Can you work these out from the model? Positions are in its coordinate system, mm. Face numbers are marked on the shaded views. A direction names the side the tool comes from. Give positions to 0.01 mm unless a question says otherwise; leave off trailing zeros. Order: outer loops, then holes, each group sorted by start corner. A loop starts at its lowest first (then second) coordinate and runs counter-clockwise, first axis right, second up. Notation, with made-up numbers: M -24.5,10.25 L 14.5,10.25 A24 ccw 14.5,33.25 Z; hole C 34.25,-16 d1. An arc over 180 degrees is marked long. One line per question, with ' | ' between items. Start each with the question number.
1) If we section it at A-A, the plane y = 7: Please give me the cut outline in (x, z), plus the area to 3 significant figures.
2) I'm going to push flat-ended pins straight in: pin 1 Ø6 at (x, y) = (-20.5, 0) entering from -Z; pin 2 Ø12 at (x, z) = (-54, -16.5) entering from +Y; pin 3 Ø6 at (y, z) = (29, -5.5) entering from +X. Where does each tip first touch, or does it pass through?
3) If we section it at B-B, the plane x = -31: Please give me the cut outline in (y, z).
4) For the marked faces 1 and 2, which set-ups out of +Z, -Z, +X, -X, +Y, -Y let a thin tool reach every point of the face, with its end or its side?
5) Please list where these lines run through material, in increasing order: line 1 along Y through (x, z) = (-44, -14.75); line 2 along Z through (x, y) = (-12.5, -12); line 3 along Y through (x, z) = (-53, -1). Write a range as [from, to].
6) If we section it at D-D, the plane x = -5: Please give me the cut outline in (y, z).
7) If we section it at C-C, the plane z = -15.25: Please give me the cut outline in (x, y).
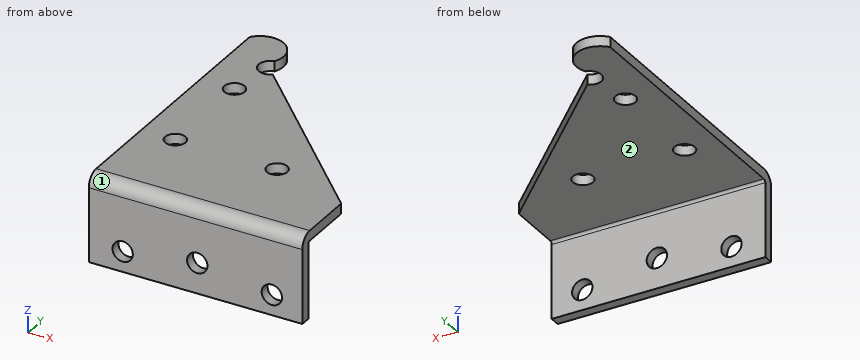
```python
from build123d import *

# Parameters (mm, degrees)
SCHIZZO2_R                           = 3
BASE_FLANGIA1_DEPTH                  = 3
PIEGATURA_START                      = -41.4
PIEGATURA_DELLO_SCHIZZO1_OUTLINE_W   = 63
PIEGATURA_DELLO_SCHIZZO1_OUTLINE_H   = 3
PIEGATURA_DELLO_SCHIZZO1_DEPTH       = 21.6634
PIEGATURA_START_2                    = -19.383939692
PIEGATURA_DELLO_SCHIZZO1_2_OUTLINE_W = 63
PIEGATURA_DELLO_SCHIZZO1_2_OUTLINE_H = 22.623356935
PIEGATURA_DELLO_SCHIZZO1_2_OUTLINE_R = 3
PIEGATURA_DELLO_SCHIZZO1_2_DEPTH     = 2.647339692
PIEGATURA_START_3                    = -19.7366
PIEGATURA_DELLO_SCHIZZO1_3_OUTLINE_W = 63
PIEGATURA_DELLO_SCHIZZO1_3_OUTLINE_H = 22.623356935
PIEGATURA_DELLO_SCHIZZO1_3_OUTLINE_R = 3
PIEGATURA_DELLO_SCHIZZO1_3_DEPTH     = 3.7366
PIEGATURA_START_4                    = -64
PIEGATURA_DELLO_SCHIZZO1_4_DEPTH     = 64


with BuildPart() as part:
    # Base-Flangia1: sheet metal written as solids
    # Schizzo2 → Base-Flangia1 (new body)
    with BuildSketch(Plane.XY):
        with BuildLine():
            Line((0, 0), (0, -41.4))
            Line((0, -41.4), (-63, -41.4))
            Line((-63, -41.4), (-63, 61.925683224))
            ThreePointArc((-63, 61.925683224), (-53.724596428, 63.490157792), (-51.266546346, 54.410582808))
            ThreePointArc((-51.266546346, 54.410582808), (-53.647048092, 49.463861618), (-48.285339065, 48.285339065))
            Line((-48.285339065, 48.285339065), (0, 0))
        make_face()
        with Locations((-53, 37)):
            Circle(SCHIZZO2_R, mode=Mode.SUBTRACT)
        with Locations((-53, 7)):
            Circle(SCHIZZO2_R, mode=Mode.SUBTRACT)
        with Locations((-23, 7)):
            Circle(SCHIZZO2_R, mode=Mode.SUBTRACT)
        with Locations((-53, -35.4)):
            Circle(SCHIZZO2_R, mode=Mode.SUBTRACT)
        with Locations((-31, -32.4)):
            Circle(SCHIZZO2_R, mode=Mode.SUBTRACT)
        with Locations((-9, -35.4)):
            Circle(SCHIZZO2_R, mode=Mode.SUBTRACT)
    extrude(amount=-BASE_FLANGIA1_DEPTH)

    # Piegatura dello schizzo1: read off the stored shape, not the designer's step
    # Piegatura dello schizzo1 outline → Piegatura dello schizzo1 (cut)
    with BuildSketch(Plane(origin=(0, 0, 0), x_dir=(1, 0, 0), z_dir=(0, 1, 0)).offset(PIEGATURA_START)):
        with Locations((-31.5, 1.5)):
            Rectangle(PIEGATURA_DELLO_SCHIZZO1_OUTLINE_W, PIEGATURA_DELLO_SCHIZZO1_OUTLINE_H)
    extrude(amount=PIEGATURA_DELLO_SCHIZZO1_DEPTH, mode=Mode.SUBTRACT)

    # Piegatura dello schizzo1 2 outline → Piegatura dello schizzo1 2 (add)
    with BuildSketch(Plane(origin=(0, 0, 0), x_dir=(1, 0, 0), z_dir=(0, 1, 0)).offset(PIEGATURA_START_2)):
        with Locations((-31.5, 14.311678468)):
            Rectangle(PIEGATURA_DELLO_SCHIZZO1_2_OUTLINE_W, PIEGATURA_DELLO_SCHIZZO1_2_OUTLINE_H)
        with Locations((-53, 19.623356935)):
            Circle(PIEGATURA_DELLO_SCHIZZO1_2_OUTLINE_R, mode=Mode.SUBTRACT)
        with Locations((-31, 16.623356935)):
            Circle(PIEGATURA_DELLO_SCHIZZO1_2_OUTLINE_R, mode=Mode.SUBTRACT)
        with Locations((-9, 19.623356935)):
            Circle(PIEGATURA_DELLO_SCHIZZO1_2_OUTLINE_R, mode=Mode.SUBTRACT)
    extrude(amount=PIEGATURA_DELLO_SCHIZZO1_2_DEPTH)

    # Piegatura dello schizzo1 3 outline → Piegatura dello schizzo1 3 (add)
    with BuildSketch(Plane(origin=(0, 0, 0), x_dir=(1, 0, 0), z_dir=(0, 1, 0)).offset(PIEGATURA_START_3)):
        with Locations((-31.5, 14.311678468)):
            Rectangle(PIEGATURA_DELLO_SCHIZZO1_3_OUTLINE_W, PIEGATURA_DELLO_SCHIZZO1_3_OUTLINE_H)
        with Locations((-53, 19.623356935)):
            Circle(PIEGATURA_DELLO_SCHIZZO1_3_OUTLINE_R, mode=Mode.SUBTRACT)
        with Locations((-31, 16.623356935)):
            Circle(PIEGATURA_DELLO_SCHIZZO1_3_OUTLINE_R, mode=Mode.SUBTRACT)
        with Locations((-9, 19.623356935)):
            Circle(PIEGATURA_DELLO_SCHIZZO1_3_OUTLINE_R, mode=Mode.SUBTRACT)
    extrude(amount=PIEGATURA_DELLO_SCHIZZO1_3_DEPTH)

    # Piegatura dello schizzo1 4 outline → Piegatura dello schizzo1 4 (cut)
    with BuildSketch(Plane.YZ.offset(PIEGATURA_START_4)):
        with BuildLine():
            ThreePointArc((-16, -3), (-16.520854855, -3.215745145), (-16.7366, -3.7366))
            Line((-16.7366, -3.7366), (-16.7366, -25.623356935))
            Line((-16.7366, -25.623356935), (-16, -25.623356935))
            Line((-16, -25.623356935), (-16, -3))
        make_face()
        with BuildLine():
            Line((-19.7366, 0), (-19.7366, -3.7366))
            ThreePointArc((-19.7366, -3.7366), (-18.642175199, -1.094424801), (-16, 0))
            Line((-16, 0), (-19.7366, 0))
        make_face()
    extrude(amount=PIEGATURA_DELLO_SCHIZZO1_4_DEPTH, mode=Mode.SUBTRACT)


solid = part.part
```
Results found:
1) outline: M -63,-3 L -56,-3 L -56,0 L -63,0 Z; M -50,-3 L -26,-3 L -26,0 L -50,0 Z; M -20,-3 L -7,-3 L -7,0 L -20,0 Z | area: 132 mm²
2) pin 1: stops at z = -3 | pin 2: stops at y = -16.74 | pin 3: stops at x = -27.34
3) outline: M -19.74,-25.62 L -16.74,-25.62 L -16.74,-19.62 L -19.74,-19.62 Z; M -19.74,-13.62 L -16.74,-13.62 L -16.74,-3.74 A0.74 cw -16,-3 L 31,-3 L 31,0 L -16,0 A3.74 ccw -19.74,-3.74 Z
4) face 1: +Z, +X, -X, -Y | face 2: -Z, +X, -X, +Y
5) line 1: y = [-19.74, -16.74] | line 2: z = [-3, 0] | line 3: y = [-18.54, 4], [10, 34], [40, 48.55], [53.45, 62.96]
6) outline: M -19.74,-25.62 L -16.74,-25.62 L -16.74,-3.74 A0.74 cw -16,-3 L 5,-3 L 5,0 L -16,0 A3.74 ccw -19.74,-3.74 Z
7) outline: M -63,-19.74 L -33.67,-19.74 L -33.67,-16.74 L -63,-16.74 Z; M -28.33,-19.74 L 0,-19.74 L 0,-16.74 L -28.33,-16.74 Z
